from build123d import *

# Parameters (mm, degrees)
SKETCH1_W           = 10
SKETCH1_H           = 10
BOSS_EXTRUDE1_DEPTH = 65
SKETCH2_W           = 30
SKETCH2_H           = 10
SKETCH2_R           = 2
BOSS_EXTRUDE2_DEPTH = 6
SKETCH3_W           = 10
SKETCH3_H           = 5
BOSS_EXTRUDE3_DEPTH = 6
SKETCH4_W           = 8
SKETCH4_H           = 16
BOSS_EXTRUDE4_DEPTH = 4
SKETCH5_W           = 6
SKETCH5_H           = 4
BOSS_EXTRUDE5_DEPTH = 10
FILLET1_START       = 2.0000001
FILLET1_DEPTH       = 2.9999999
FILLET1_START_2     = -5
FILLET1_2_DEPTH     = 2.999999286
FILLET1_START_3     = -2.000000714
FILLET1_3_DEPTH     = 4.000000814
FILLET1_4_DEPTH     = 10
FILLET1_5_OUTLINE_R = 2
FILLET1_5_DEPTH     = 11
SKETCH6_R           = 3
CUT_EXTRUDE1_DEPTH  = 69
FILLET2_R           = 8


with BuildPart() as part:
    # Sketch1 → Boss-Extrude1 (new body)
    with BuildSketch(Plane.XY):
        Rectangle(SKETCH1_W, SKETCH1_H)
    extrude(amount=BOSS_EXTRUDE1_DEPTH)

    # Sketch2 → Boss-Extrude2 (add)
    with BuildSketch(Plane(origin=(0, 0, 0), x_dir=(-1, 0, 0), z_dir=(0, 0, -1))):
        Rectangle(SKETCH2_W, SKETCH2_H)
        with Locations((-10, 0)):
            Circle(SKETCH2_R, mode=Mode.SUBTRACT)
        with Locations((10, 0)):
            Circle(SKETCH2_R, mode=Mode.SUBTRACT)
    extrude(amount=BOSS_EXTRUDE2_DEPTH)

    # Sketch3 → Boss-Extrude3 (add)
    with BuildSketch(Plane(origin=(0, 5, 0), x_dir=(1, 0, 0), z_dir=(0, 1, 0))):
        with Locations((0, -62.5)):
            Rectangle(SKETCH3_W, SKETCH3_H)
    extrude(amount=BOSS_EXTRUDE3_DEPTH)

    # Sketch4 → Boss-Extrude4 (add)
    with BuildSketch(Plane.XY.offset(65)):
        with Locations((0, 3)):
            Rectangle(SKETCH4_W, SKETCH4_H)
    extrude(amount=BOSS_EXTRUDE4_DEPTH)

    # Sketch5 → Boss-Extrude5 (add)
    with BuildSketch(Plane.XY.offset(69)):
        with Locations((0, 9)):
            Rectangle(SKETCH5_W, SKETCH5_H)
    extrude(amount=BOSS_EXTRUDE5_DEPTH)

    # Fillet1: read off the stored shape, not the designer's step
    # Fillet1 outline → Fillet1 (add)
    with BuildSketch(Plane(origin=(0, 0, 0), x_dir=(1, 0, 0), z_dir=(0, 1, 0)).offset(FILLET1_START)):
        with BuildLine():
            ThreePointArc((-15, 0), (-7.928932188, -2.928932188), (-5, -10))
            Line((-5, -10), (-5, 0))
            Line((-5, 0), (-15, 0))
        make_face()
        with BuildLine():
            Line((5, 0), (5, -10))
            ThreePointArc((5, -10), (7.928932188, -2.928932188), (15, 0))
            Line((15, 0), (5, 0))
        make_face()
    extrude(amount=FILLET1_DEPTH)

    # Fillet1 2 outline → Fillet1 2 (add)
    with BuildSketch(Plane(origin=(0, 0, 0), x_dir=(1, 0, 0), z_dir=(0, 1, 0)).offset(FILLET1_START_2)):
        with BuildLine():
            ThreePointArc((-15, 0), (-7.928932188, -2.928932188), (-5, -10))
            Line((-5, -10), (-5, 0))
            Line((-5, 0), (-15, 0))
        make_face()
        with BuildLine():
            Line((5, 0), (5, -10))
            ThreePointArc((5, -10), (7.928932188, -2.928932188), (15, 0))
            Line((15, 0), (5, 0))
        make_face()
    extrude(amount=FILLET1_2_DEPTH)

    # Fillet1 3 outline → Fillet1 3 (add)
    with BuildSketch(Plane(origin=(0, 0, 0), x_dir=(1, 0, 0), z_dir=(0, 1, 0)).offset(FILLET1_START_3)):
        with BuildLine():
            ThreePointArc((-15, 0), (-7.928932188, -2.928932188), (-5, -10))
            Line((-5, -10), (-5, 0))
            Line((-5, 0), (-15, 0))
        make_face()
        with BuildLine():
            Line((5, 0), (5, -10))
            ThreePointArc((5, -10), (7.928932188, -2.928932188), (15, 0))
            Line((15, 0), (5, 0))
        make_face()
    extrude(amount=FILLET1_3_DEPTH)

    # Fillet1 4 outline → Fillet1 4 (add)
    with BuildSketch(Plane.YZ.offset(FILLET1_START_2)):
        with BuildLine():
            ThreePointArc((5, 50.83484861), (6.633399735, 56.312074185), (11, 60))
            Line((11, 60), (5, 60))
            Line((5, 60), (5, 50.83484861))
        make_face()
    extrude(amount=FILLET1_4_DEPTH)

    # Fillet1 5 outline → Fillet1 5 (cut)
    with BuildSketch(Plane.XY):
        with Locations((10, 0)):
            Circle(FILLET1_5_OUTLINE_R)
        with Locations((-10, 0)):
            Circle(FILLET1_5_OUTLINE_R)
    extrude(amount=FILLET1_5_DEPTH, mode=Mode.SUBTRACT)

    # Sketch6 → Cut-Extrude1 (cut)
    with BuildSketch(Plane.XY.offset(69)):
        with Locations((-10, 0)):
            Circle(SKETCH6_R)
        with Locations((10, 0)):
            Circle(SKETCH6_R)
    extrude(amount=-CUT_EXTRUDE1_DEPTH, mode=Mode.SUBTRACT)

    # Fillet2
    # the kernel refuses this fillet: 8 mm, written as the material it adds along each edge
    with BuildSketch(Plane(origin=(4, -5, 65), x_dir=(1, 0, 0), z_dir=(0, 1, 0))) as fillet2_piece_1:
        with BuildLine():
            CenterArc((8, -3.872983346), FILLET2_R, 151.044975628, 28.955024372)
            Line((0, -3.872983346), (0, 0))
            Line((0, 0), (1, 0))
        make_face()
    extrude(amount=16)
    with BuildSketch(Plane(origin=(-4, 11, 65), x_dir=(0, 0, 1), z_dir=(0, -1, 0))) as fillet2_piece_2:
        with BuildLine():
            CenterArc((3.872983346, 8), FILLET2_R, 241.044975628, 28.955024372)
            Line((0, 1), (0, 0))
            Line((0, 0), (3.872983346, 0))
        make_face()
    extrude(amount=16)


solid = part.part
Model file for the job. Use its own axes, mm. A direction names the side the tool comes from. Round coordinates to 2 decimals unless told otherwise and drop trailing zeros. Loops run counter-clockwise (first coordinate to the right, second up) from the corner with the lowest first, then second, coordinate; pieces in that order, holes last.
1. Mould opens along X. For faces 1 (the cylindrical face through (6.75, -0.07, 4.35)), 2 (the cylindrical face through (-7.14, 0.9, 1.58)), 3 (the flat face through (0, 11, 68)) say: +X half, -X half, draft (parallel to the pull), parting line (faces both ways), or undercut.
Check values:
face 1: +X half
face 2: undercut
face 3: draft
2. Band-saw the part on D-D, the plane y = 10. List the corners of the cut face in (x, z), and give its area (3 significant figures).
Check values:
outline: (-5, 59.5) - (5, 59.5) - (5, 65) arc R8 cw to (4, 68.87) - (4, 69) - (3, 69) - (3, 79) - (-3, 79) - (-3, 69) - (-4, 69) - (-4, 68.87) arc R8 cw to (-5, 65) - close
area: 150 mm2
3. Band-saw the part on B-B, the plane x = 10. List the corners of the cut face in (y, z).
Check values:
outline: (-5, -6) - (-2, -6) - (-2, 0) - (-3, 0) - (-3, 1.34) - (-5, 1.34) - close; (2, -6) - (5, -6) - (5, 1.34) - (3, 1.34) - (3, 0) - (2, 0) - close
4. Band-saw the part on C-C, the plane z = 36. List the corners of the cut face in (x, y).
Check values:
outline: (-5, -5) - (5, -5) - (5, 5) - (-5, 5) - close
5. Tool access for faces 4 (the flat face through (-5, 1, 38)), 5 (the flat face through (3, 9, 74)), 6 (the flat face through (0, 7, 74)), 7 (the flat face through (0, 5, 16)): list every direction of +Z, -Z, +X, -X, +Y, -Y with a clear straight run to the whole face (end or side of a thin tool).
Check values:
face 4: +Z, -X, +Y, -Y
face 5: +Z, +X, +Y, -Y
face 6: +Z, +X, -X, -Y
face 7: -Z, +X, -X, +Y
6. Wall check: probe 1 along Y at (x, z) = (10, -3); probe 2 along Y at (x, z) = (-10, 1); probe 3 along X at (y, z) = (1.75, 64). Give the ranges that are in metal, low to high.
Check values:
probe 1: y = -5 to -2, 2 to 5
probe 2: y = -5 to -3, 3 to 5
probe 3: x = -5 to 5
7. Drop flat-ended pins along their axis: P1, Ø1, axis at y = 5, z = 68.5, coming from the -X side; P2, Ø6.5, axis at x = 10, y = 0, coming from the +Z side; P3, Ø3, axis at x = 1.5, z = 35, coming from the +Y side. Give the stop position or say it passes through.
Check values:
P1: stops at x = -4.05
P2: stops at z = 4.35
P3: stops at y = 5
8. Band-saw the part on A-A, the plane y = 0. List the corners of the cut face in (x, z).
Check values:
outline: (-15, -6) - (-12, -6) - (-12, 0) - (-13, 0) - (-13, 0.2) arc R10 cw to (-15, 0) - close; (-8, -6) - (8, -6) - (8, 0) - (7, 0) - (7, 4) arc R10 cw to (5, 10) - (5, 65) arc R8 cw to (4, 68.87) - (4, 69) - (-4, 69) - (-4, 68.87) arc R8 cw to (-5, 65) - (-5, 10) arc R10 cw to (-7, 4) - (-7, 0) - (-8, 0) - close; (12, -6) - (15, -6) - (15, 0) arc R10 cw to (13, 0.2) - (13, 0) - (12, 0) - close
